Autodesk Inventor part; units mm, degrees
ref_plane "Work Plane1" through (0, 0, -15) normal (0, 0, 1) x (1, 0, 0)
ref_plane "YZ Plane" through (0, 0, 0) normal (1, 0, 0) x (0, 1, 0)
ref_plane "XZ Plane" through (0, 0, 0) normal (0, 1, 0) x (-1, 0, 0)
sketch "Sketch1" plane through (0, 0, 0) normal (0, 0, 1) x (1, 0, 0)
  line L0 (0, 0) -> (25, 0)
  line L1 (25, 0) -> (25, 40)
  line L2 (25, 40) -> (0, 40)
  line L3 (0, 40) -> (0, 0)
  dimension "d1" = 25
  dimension "d2" = 40
  dimension "d3" = 25
extrude "Extrusion1" add sketch "Sketch1" against normal blind 30
sketch "Sketch2" plane through (25, 0, 0) normal (1, 0, 0) x (0, 0, -1)
  line L0 (0, 0) -> (30, 0)
  circle A0 centre (15, 6.56) radius 2.46
extrude "Extrusion2" cut sketch "Sketch2" against normal blind 30
sketch "Sketch3" plane through (0, 0, 0) normal (-1, 0, 0) x (0, 0, 1)
  line L0 (0, 0) -> (-30, 0)
  line L1 (-25.05, 0) -> (-4.95, 0)
  line L2 (-4.95, 0) -> (-4.95, 33.12)
  line L3 (-4.95, 33.12) -> (-25.05, 33.12)
  line L4 (-25.05, 33.12) -> (-25.05, 0)
  dimension "d11" = 20.1
extrude "Extrusion3" cut sketch "Sketch3" against normal blind 20
sketch "Sketch4" plane through (0, 0, 0) normal (0, -1, 0) x (1, 0, 0)
  line L0 (20, -4.95) -> (20, -25.05)
  line L1 (20, -15) -> (25, -15)
  line L2 (25, 0) -> (25, -30)
  line L3 (20, -8.025) -> (25, -8.025)
  line L4 (25, -8.025) -> (25, -21.975)
  line L5 (25, -21.975) -> (20, -21.975)
  line L6 (20, -21.975) -> (20, -8.025)
  line L7 (20, -8.025) -> (25, -21.975) construction
  line L8 (25, -8.025) -> (20, -21.975) construction
  line L9 (25, -12.54) -> (25, -17.46)
  point P0 (0, 0)
  point P1 (22.5, -15)
  dimension "d14" = 13.95
extrude "Extrusion4" add sketch "Sketch4" along normal blind 15
sketch "Sketch5" plane through (20, 0, 0) normal (-1, 0, 0) x (0, 0, 1)
  circle A0 centre (-15, 6.56) radius 2.46
  circle A1 centre (-15, 6.56) radius 4.7025
  circle A2 centre (-15, 6.56) radius 2.46
  circle A3 centre (-15, 6.56) radius 2.46
  point P0 (0, 0)
  dimension "d17" = 9.405
extrude "Extrusion5" cut sketch "Sketch5" against normal blind 2.1
sketch "Sketch6" plane through (25, 0, 0) normal (1, 0, 0) x (0, 0, -1)
  circle A0 centre (15, 6.56) radius 4.7025
  line L0 (15, 6.56) -> (15, 23.56)
  circle A1 centre (15, 23.56) radius 2.46
  point P0 (0, 0)
  dimension "d20" = 17
  dimension "d21" = 4.92
extrude "Extrusion6" cut sketch "Sketch6" against normal blind 10 contours A1
sketch "Sketch7" plane through (20, 0, 0) normal (-1, 0, 0) x (0, 0, 1)
  circle A0 centre (-15, 23.56) radius 2.46
  circle A1 centre (-15, 23.56) radius 4.7025
  point P0 (0, 0)
  dimension "d24" = 9.405
extrude "Extrusion7" cut sketch "Sketch7" against normal blind 2.1
sketch "Sketch9" plane through (25, 0, 0) normal (1, 0, 0) x (0, 0, -1)
  circle A0 centre (15, 6.56) radius 2.46
  circle A1 centre (15, 6.56) radius 2.46
  circle A2 centre (15, 23.56) radius 2.46
  circle A3 centre (15, 23.56) radius 2.46
  line L0 (30, 40) -> (30, 0)
  line L1 (30, 0) -> (30, 40)
  line L2 (30, 40) -> (0, 40)
  line L3 (0, 40) -> (0, 0)
  line L4 (0, 0) -> (8.025, 0)
  line L5 (21.975, 0) -> (21.975, -15)
  line L6 (21.975, -15) -> (8.025, -15)
  line L7 (8.025, -15) -> (8.025, 0)
  line L8 (0, 0) -> (8.025, 0)
  line L9 (21.975, 0) -> (30, 0)
extrude "Extrusion8" add sketch "Sketch9" along normal blind 5
sketch "Sketch10" plane through (0, 40, 0) normal (0, 1, 0) x (1, 0, 0)
  line L0 (0, 30) -> (30, 30)
  line L1 (30, 0) -> (0, 0)
  line L2 (0, 30) -> (30, 30)
  line L3 (30, 30) -> (30, 0)
  line L4 (30, 0) -> (0, 0)
  line L5 (0, 0) -> (0, 30)
extrude "Extrusion9" add sketch "Sketch10" along normal blind 30
sketch "Sketch12" plane through (30, 0, 0) normal (1, 0, 0) x (0, 0, -1)
  circle A0 centre (15, 6.56) radius 2.46
  line L0 (15, 6.56) -> (15, 15.06)
  circle A1 centre (15, 15.06) radius 2.525
  point P0 (0, 0)
  dimension "d31" = 8.5
  dimension "d33" = 5.05
extrude "Extrusion10" cut sketch "Sketch12" against normal blind 30 contours A1
sketch "Sketch14" plane through (0, 0, 0) normal (0, 0, 1) x (1, 0, 0)
  line L0 (30, 70) -> (0, 70)
  line L1 (0, 100) -> (-8, 100)
  line L2 (30, 0) -> (30, 70)
  line L3 (30, 118) -> (30, 70)
  line L4 (30, 105) -> (30, 100)
  line L5 (-2, 134) -> (-8, 136)
  line L6 (-2, 134) -> (4, 118)
  line L7 (-2, 102) -> (-8, 100)
  line L8 (-2, 102) -> (4, 118)
  line L9 (0, 70) -> (30, 70)
  line L10 (0, 70) -> (0, 100)
  line L11 (15, 136) -> (30, 118)
  line L12 (-8, 136) -> (15, 136)
  point P0 (0, 0)
  dimension "d47" = 30
extrude "Extrusion12" add sketch "Sketch14" against normal blind 30
sketch "Sketch15" plane through (0, 0, -25.05) normal (-1, 0, 0) x (0, 0, 1)
  line L0 (0, 33.12) -> (20.1, 33.12)
  line L1 (20.1, 33.12) -> (20.1, 0)
  line L2 (0, 33.12) -> (20.1, 33.12)
  line L3 (20.1, 33.12) -> (20.1, 31.1)
  line L4 (20.1, 31.1) -> (0, 31.1)
  line L5 (0, 31.1) -> (0, 33.12)
  point P0 (25.05, 0)
  dimension "d57" = 2.02
extrude "Extrusion13" add sketch "Sketch15" against normal blind 20
sketch "Sketch23" plane through (0, 0, 0) normal (0, 0, 1) x (1, 0, 0)
  line L0 (0, 100) -> (-8, 100)
  line L1 (-8, 100) -> (-2, 102)
  line L2 (-8, 100) -> (-2, 102)
  line L3 (-2, 102) -> (4, 118)
  line L4 (-2, 102) -> (4, 118)
  line L5 (-2, 134) -> (4, 118)
  line L6 (4, 118) -> (-2, 134)
  line L7 (-2, 134) -> (-8, 136)
  line L8 (-2, 134) -> (-8, 136)
  line L9 (-8, 136) -> (15, 136)
  line L10 (-8, 136) -> (15, 136)
  line L11 (30, 118) -> (15, 136)
  line L12 (15, 136) -> (30, 118)
  line L13 (30, 118) -> (30, 93)
  line L14 (30, 0) -> (30, 118)
  line L15 (30, 93) -> (0, 93)
  line L16 (0, 93) -> (0, 100)
  line L17 (-8, 100) -> (0, 100)
  point P0 (0, 0)
  dimension "d85" = 25
extrude "Extrusion14" add sketch "Sketch23" along normal blind 30
ref_plane "Work Plane1" through (0, 0, -15) normal (0, 0, 1) x (1, 0, 0)
mirror "Mirror1" about plane through (0, 0, -15) normal (0, 0, 1) of "Extrusion14"
properties part number "32mm_x_90mm"
Verification items for the finished model (mm, model axes). A direction names the side the tool comes from. Give positions to 0.01 mm unless a question says otherwise; leave off trailing zeros. Loops run counter-clockwise (first coordinate to the right, second up) from the corner with the lowest first, then second, coordinate; pieces in that order, holes last. Notation, with made-up numbers: M -32.75,56.25 L 18.25,56.25 A8 cw 18.25,68.25 Z; hole C 82,39 d6. An arc over 180 degrees is marked long. One line per question, with ' | ' between items.
Item 1: Section check D-D, the plane x = 10. Record the cut outline in (y, z), plus the area to 3 significant figures.
Completed:
outline: M 0,-30 L 93,-30 L 93,-60 L 136,-60 L 136,30 L 93,30 L 93,0 L 0,0 L 0,-4.95 L 31.1,-4.95 L 31.1,-25.05 L 0,-25.05 Z | area: 6,030 mm^2
Item 2: Draft check along Z on faces 1 (the face through (25.995, 7.502, -17.272)), 2 (the face through (25, -7, -21.975)), 3 (the face through (25, -15, -15)). Enter one of: +Z half, -Z half, draft (parallel to the pull), parting line (faces both ways), or undercut.
Completed:
face 1: undercut | face 2: -Z half | face 3: draft
Item 3: Section check B-B, the plane z = -15. State how many separate pieces and enclosed holes the cut face has, plus the area to 3 significant figures.
Completed:
separate pieces: 4 | enclosed holes: 0 | area: 3,290 mm^2
Item 4: Thickness scan on line 1 (Z direction, x = 26.25, y = 15.06) (3 decimals); line 2 (Z direction, x = 2, y = 6.5); line 3 (Y direction, x = 9, z = -0.5). Record the ranges inside material, lowest first. Write a range as [from, to].
Completed:
line 1: z = [-30, -17.525], [-12.475, 0] | line 2: z = [-30, -25.05], [-4.95, 0] | line 3: y = [0, 136]
Item 5: Section check C-C, the plane x = 24. Record the cut outline in (y, z) (3 decimals), plus the area to 3 significant figures.
Completed:
outline: M -15,-21.975 L 0,-21.975 L 0,-30 L 93,-30 L 93,-60 L 125.2,-60 L 125.2,30 L 93,30 L 93,0 L 0,0 L 0,-8.025 L -15,-8.025 Z; hole C 6.56,-15 d4.92; hole C 15.06,-15 d5.05; hole C 23.56,-15 d4.92 | area: 5,840 mm^2
Item 6: Section check A-A, the plane y = 23.56. Record the cut outline in (x, z).
Completed:
outline: M 0,-30 L 30,-30 L 30,-17.46 L 22.1,-17.46 L 22.1,-19.7 L 20,-19.7 L 20,-25.05 L 0,-25.05 Z; M 0,-4.95 L 20,-4.95 L 20,-10.3 L 22.1,-10.3 L 22.1,-12.54 L 30,-12.54 L 30,0 L 0,0 Z
Item 7: Depth check by flat-ended pin: P1, Ø6, axis at x = 19.5, z = -5, coming from the +Y side; P2, Ø5.5, axis at y = 23.56, z = -15, coming from the -X side; P3, Ø22, axis at x = 5, y = 22, coming from the +Z side; P4, Ø4.5, axis at y = 6.56, z = -15, coming from the -X side. Enter the tip coordinate at first touch or a pass-through.
Completed:
P1: stops at y = 134.2 | P2: stops at x = 22.1 | P3: stops at z = 0 | P4: passes through
Item 8: Tool access check on faces 4 (the face through (1, 110, -14)), 5 (the face through (0, 65, -15)), 6 (the face through (15, 0, -3)). Record the directions out of +Z, -Z, +X, -X, +Y, -Y that give a thin tool (end or side, any length) a straight path to the whole face; none if there is none.
Completed:
face 4: +Z, -Z, -X | face 5: +Z, -Z, -X, -Y | face 6: +Z, +X, -X, -Y
